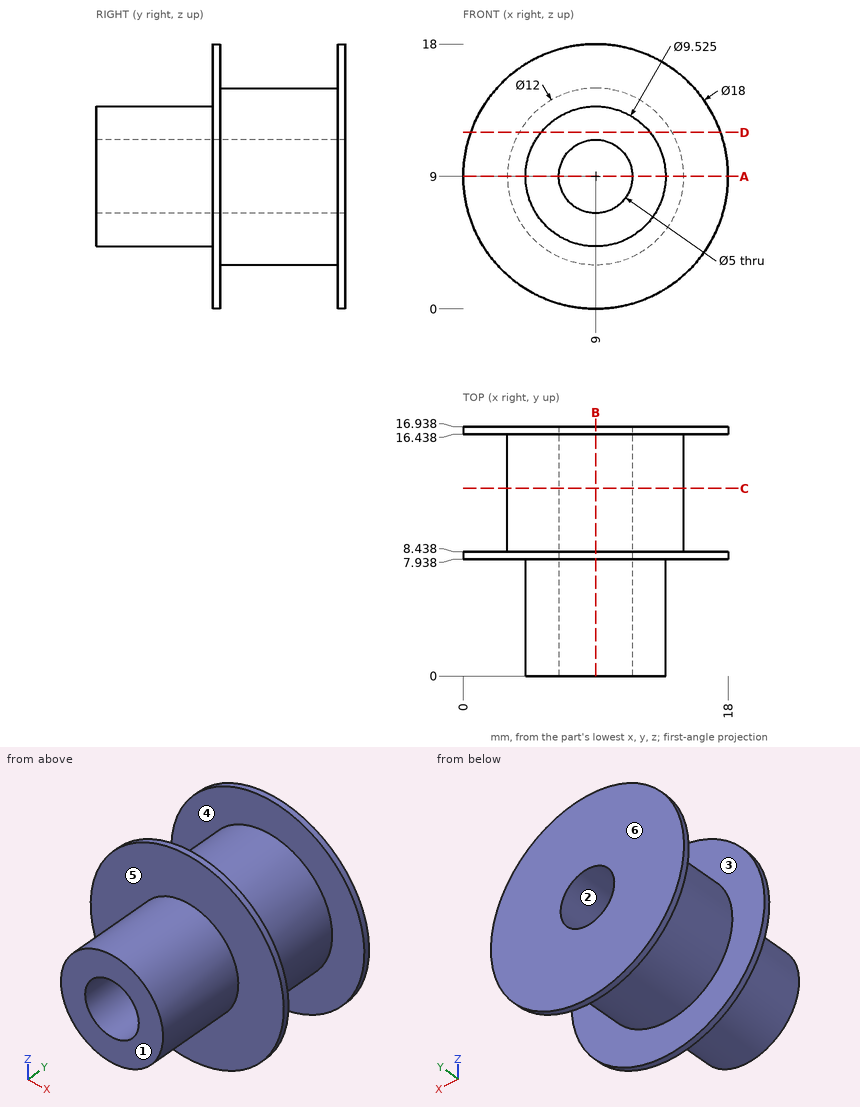
Can you work these out from the drawing? Everything is in mm from the part's minimum corner. A direction names the side the tool comes from. Give positions to 0.01 mm unless a question says otherwise; leave off trailing zeros. Write each loop counter-clockwise with the first axis right and the second up, starting at its lowest first coordinate (ties: lowest second). Pieces come first, ordered by that corner, then holes. Notation, with made-up numbers: M -25,64 L 18,64 A19 ccw 18,75 Z; hole C 77.5,28 d9. An arc over 180 degrees is marked long. Answer in a Markdown table with one row per item. Add a question column.
Item 1: For pin 1 Ø6 at (x, y) = (14.5, 13) entering from -Z (1 decimal); pin 2 Ø3 at (y, z) = (12, 4.5) entering from -X (1 decimal); pin 3 Ø5 at (x, y) = (9.5, 5) entering from +Z, each with a flat end and sliding along its axis, tell me the tip position at first contact or that it passes through.
Item 2: Imagine slicing it at B-B, the plane x = 9. Write out the boundary of the cut face in (y, z), plus the area to 3 significant figures.
Item 3: On a 3-axis mill with a long thin cutter (end or side, diameter ignored), from which of +Z, -Z, +X, -X, +Y, -Y can I reach the whole of each face in a straight line? I mean the marked faces 4, 5 and 6. Say none if no direction works.
Item 4: Imagine slicing it at C-C, the plane y = 12.75. Write out the boundary of the cut face in (x, z).
Item 5: We'd pull the mould along Y, two halves only. Please class the marked faces 1, 2 and 3: released by +Y, released by -Y, zero draft, split by the parting line, or undercut.
Item 6: Imagine slicing it at D-D, the plane z = 12. Write out the boundary of the cut face in (x, y) (1 decimal).
Item 7: Imagine slicing it at A-A, the plane z = 9. Write out the boundary of the cut face in (x, y).
Item 8: Please list where these lines run through material, in increasing order: L1, parallel to Y at x = 12, z = 15; L2, parallel to X at y = 4.25, z = 9; L3, parallel to X at y = 12.25, z = 9.
Evaluation:
| question | item | result |
|---|---|---|
| 1 | pin 1 | stops at z = 3.5 |
| 1 | pin 2 | stops at x = 3.8 |
| 1 | pin 3 | stops at z = 13.76 |
| 2 | outline | M 0,4.24 L 7.94,4.24 L 7.94,0 L 8.44,0 L 8.44,3 L 16.44,3 L 16.44,0 L 16.94,0 L 16.94,6.5 L 0,6.5 Z; M 0,11.5 L 16.94,11.5 L 16.94,18 L 16.44,18 L 16.44,15 L 8.44,15 L 8.44,18 L 7.94,18 L 7.94,13.76 L 0,13.76 Z |
| 2 | area | 105 mm² |
| 3 | face 4 | none |
| 3 | face 5 | -Y |
| 3 | face 6 | +Z, -Z, +X, -X, +Y |
| 4 | outline | C 9,9 d12; hole C 9,9 d5 |
| 5 | face 1 | released by -Y |
| 5 | face 2 | zero draft |
| 5 | face 3 | undercut |
| 6 | outline | M 0.5,7.9 L 5.3,7.9 L 5.3,0 L 12.7,0 L 12.7,7.9 L 17.5,7.9 L 17.5,8.4 L 14.2,8.4 L 14.2,16.4 L 17.5,16.4 L 17.5,16.9 L 0.5,16.9 L 0.5,16.4 L 3.8,16.4 L 3.8,8.4 L 0.5,8.4 Z |
| 7 | outline | M 0,7.94 L 4.24,7.94 L 4.24,0 L 6.5,0 L 6.5,16.94 L 0,16.94 L 0,16.44 L 3,16.44 L 3,8.44 L 0,8.44 Z; M 11.5,0 L 13.76,0 L 13.76,7.94 L 18,7.94 L 18,8.44 L 15,8.44 L 15,16.44 L 18,16.44 L 18,16.94 L 11.5,16.94 Z |
| 8 | L1 | y = 7.94 to 8.44, 16.44 to 16.94 |
| 8 | L2 | x = 4.24 to 6.5, 11.5 to 13.76 |
| 8 | L3 | x = 3 to 6.5, 11.5 to 15 |
